Could you check a few things on this model? Use its own coordinates, in mm. Coordinates: 2 decimals unless noted, no trailing zeros. Loops run counter-clockwise (first coordinate to the right, second up) from the corner with the lowest first, then second, coordinate; pieces in that order, holes last. Notation, with made-up numbers: M 14,48 L 21,48 A21 ccw 21,85 Z; hole C 78.5,-34 d6. An arc over 180 degrees is marked long. Write each question's results on one line, items separated by ' | '.
```python
from build123d import *

# Parameters (mm, degrees)
SKETCH1_R           = 5.08
SKETCH1_R_2         = 2.54
BOSS_EXTRUDE1_DEPTH = 2.667
CHAMFER3_SIZE       = 2.5146
CHAMFER3_SIZE2      = 1.172577237
SKETCH3_R           = 2.794
SKETCH3_R_2         = 2.54
BOSS_EXTRUDE2_DEPTH = 0.381
CHAMFER1_SIZE       = 2.286
CHAMFER1_SIZE_2     = 0.362066831
FILLET4_R           = 1.27


with BuildPart() as part:
    # Sketch1 → Boss-Extrude1 (new body)
    with BuildSketch(Plane(origin=(0, 0, 0), x_dir=(1, 0, 0), z_dir=(0, 1, 0))):
        with Locations(Location((0, 0, 0), (0, 0, 270))):
            Circle(SKETCH1_R)
        with Locations(Location((0, 0, 0), (0, 0, 270))):
            Circle(SKETCH1_R_2, mode=Mode.SUBTRACT)
    extrude(amount=BOSS_EXTRUDE1_DEPTH)

    # Chamfer3
    chamfer3_edges = [part.edges().sort_by_distance(p)[0] for p in [
        (0, 0, -5.08),
    ]]
    chamfer3_side = [part.faces().sort_by_distance(p)[0] for p in [
        (0, 0, -4.936315902),
    ]]
    chamfer(chamfer3_edges, length=CHAMFER3_SIZE, length2=CHAMFER3_SIZE2, reference=chamfer3_side[0])

    # Mirror4: part across plane


with BuildPart() as part_1:
    add(part.part)
    add(part.part.mirror(Plane.ZX))

    # Sketch3 → Boss-Extrude2 (add)
    with BuildSketch(Plane(origin=(0, 2.667, 0), x_dir=(1, 0, 0), z_dir=(0, 1, 0))):
        with Locations(Location((0, 0, 0), (0, 0, 90))):
            Circle(SKETCH3_R)
        with Locations(Location((0, 0, 0), (0, 0, 270))):
            Circle(SKETCH3_R_2, mode=Mode.SUBTRACT)
    extrude(amount=BOSS_EXTRUDE2_DEPTH)

    # Chamfer1
    # the kernel refuses this chamfer: 2.286, 0.362066831 mm, written as the material it adds along each edge
    with BuildSketch(Plane(origin=(0, 2.667, 0), x_dir=(0, 0, -1), z_dir=(1, 0, 0))) as chamfer1_piece_1_section:
        Polygon((2.794 + CHAMFER1_SIZE, 0), (2.794, CHAMFER1_SIZE_2 * 0.999999998845), (2.794, 0), align=None)
    chamfer1_piece_1 = revolve(axis=Axis((0, 2.667, 0), (0, 1, 0)), mode=Mode.PRIVATE)
    chamfer1_piece_1 = chamfer1_piece_1 & Plane(origin=(0, 2.832338602, 0), x_dir=(0, 0, 1), z_dir=(0, -1, 0)) * Cylinder(5.08, 21, mode=Mode.PRIVATE)
    add(chamfer1_piece_1)

    # Mirror5: part across plane


with BuildPart() as part_2:
    add(part_1.part)
    add(part_1.part.mirror(Plane(origin=(0, -2.667, 0), x_dir=(0, 0, 1), z_dir=(0, -1, 0))))

    # Fillet4
    fillet4_edges = [part_2.edges().sort_by_distance(p)[0] for p in [
        (0, 0, -2.5654),
        (0, -5.334, -2.5654),
    ]]
    fillet(fillet4_edges, radius=FILLET4_R)


solid = part_2.part
```
(1) Imagine slicing it at A-A, the plane y = -2. List the corners of the cut face in (x, z) for me.
Reported:
outline: C 0,0 d10.16; hole C 0,0 d5.08
(2) Please list where these lines run through material, in increasing order: probe 1 along X at (y, z) = (-2.75, 0); probe 2 along Y at (x, z) = (3.25, -3.5) (3 decimals); probe 3 along Y at (x, z) = (-4, 2.25). Write a range as from..to.
Reported:
probe 1: x = -5.08..-2.54, 2.54..5.08 | probe 2: y = -8.049..-6.325, -4.343..-0.991, 0.991..2.715 | probe 3: y = -8.08..-6.14, -4.53..-0.81, 0.81..2.74
(3) Imagine slicing it at B-B, the plane x = 4.75. State how many separate pieces and enclosed holes the cut face has, and give its area (3 significant figures).
Reported:
separate pieces: 3 | enclosed holes: 0 | area: 23.6 mm2
(4) Will these pins go through, and if not, where does the flat tip stop? P1, Ø1, axis at x = 3.5, y = -1, coming from the -Z side; P2, Ø2, axis at x = -2.5, y = 0, coming from the -Z side; P3, Ø6, axis at x = 3, z = -1.5, coming from the +Y side; P4, Ø1, axis at x = -2, y = 0, coming from the -Z side.
Reported:
P1: stops at z = -4.08 | P2: stops at z = -4.2 | P3: stops at y = 3.05 | P4: stops at z = -4.03
